from build123d import *

# Parameters (mm, degrees)
OHGC_BASE_DEPTH  = 2.54
SKETCH7_R        = 1.27
SCREWHOLES_DEPTH = 3.54


with BuildPart() as part:
    # Sketch2 → OHGC BASE (new body)
    with BuildSketch(Plane(origin=(0, 0, 0), x_dir=(1, 0, 0), z_dir=(0, 1, 0))):
        with BuildLine():
            Line((12.7, 0), (25.4, 0))
            ThreePointArc((25.4, 0), (34.380256121, 3.719743879), (38.1, 12.7))
            Line((38.1, 12.7), (38.1, 38.1))
            ThreePointArc((38.1, 38.1), (38.996434372, 41.352863652), (41.432636832, 43.68730879))
            Line((41.432636832, 43.68730879), (69.022459682, 58.586881809))
            ThreePointArc((69.022459682, 58.586881809), (73.920701901, 62.034864891), (77.875264971, 66.534064274))
            Line((77.875264971, 66.534064274), (81.475778144, 71.764628765))
            ThreePointArc((81.475778144, 71.764628765), (85.749269843, 82.951996559), (84.42171275, 94.853993098))
            Line((84.42171275, 94.853993098), (66.518139685, 144.04365582))
            ThreePointArc((66.518139685, 144.04365582), (61.868464143, 150.103230962), (54.584043401, 152.4))
            Line((54.584043401, 152.4), (6.35, 152.4))
            ThreePointArc((6.35, 152.4), (1.859871939, 150.540128061), (0, 146.05))
            Line((0, 146.05), (0, 12.7))
            ThreePointArc((0, 12.7), (3.719743879, 3.719743879), (12.7, 0))
        make_face()
    extrude(amount=OHGC_BASE_DEPTH)

    # Sketch7 → Screwholes (cut, through all)
    with BuildSketch(Plane(origin=(0, 0, 0), x_dir=(1, 0, 0), z_dir=(0, 1, 0))):
        with Locations((3.302, 149.098)):
            Circle(SKETCH7_R)
        with Locations((60.719962059, 148.463)):
            Circle(SKETCH7_R)
        with Locations((83.655901234, 83.21908607)):
            Circle(SKETCH7_R)
        with Locations((19.05, 22.352)):
            Circle(SKETCH7_R)
        with Locations((19.05, 2.032)):
            Circle(SKETCH7_R)
    extrude(amount=SCREWHOLES_DEPTH, mode=Mode.SUBTRACT)


solid = part.part
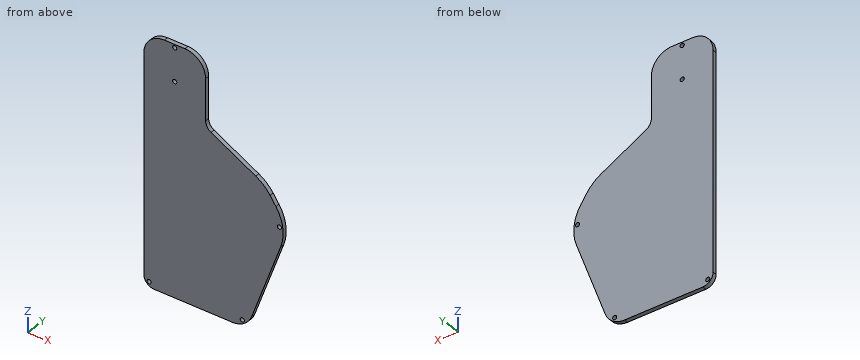
Geometry check sheet. Reference: the model listing, model coordinates, mm. Give positions to 0.01 mm unless a question says otherwise; leave off trailing zeros. Loops run counter-clockwise (first coordinate to the right, second up) from the corner with the lowest first, then second, coordinate; pieces in that order, holes last. Notation, with made-up numbers: (28.25, 60.25) -> (74.25, 60.25) arc R26 cw to (74.25, 95.25) -> close; hole circle Ø4 at (2, 79.25). An arc over 180 degrees is marked (long way). Answer in a Markdown table with one row per item. Add a question column.
1) Gauge pin test, flat end, axial feed: P1, Ø1, axis at x = 58.5, y = 2, coming from the -Z side. Record the tip position at first contact, or that the pin passes through.
2) Cross-section at C-C on x = 45.5. Record the boundary of the cut face in (y, z).
3) Cross-section at B-B on z = -142. Record the boundary of the cut face in (x, y), and give its area (3 significant figures).
4) Cross-section at A-A on y = 0.8. Record the boundary of the cut face in (x, z), and give its area (3 significant figures).
5) Material ranges on probe 1 along Z at (x, y) = (19.05, 2.05); probe 2 along X at (y, z) = (0.45, -13.5); probe 3 along Z at (x, y) = (18, 2.1), recorded low to high. Write a range as from..to.
Outcome:
| question | item | result |
|---|---|---|
| 1 | P1 | stops at z = -151.93 |
| 2 | outline | (0, -152.4) -> (2.54, -152.4) -> (2.54, -45.88) -> (0, -45.88) -> close |
| 3 | outline | (0, 0) -> (67.26, 0) -> (67.26, 2.54) -> (0, 2.54) -> close |
| 3 | area | 171 mm^2 |
| 4 | outline | (0, -146.05) arc R6.35 ccw to (6.35, -152.4) -> (54.58, -152.4) arc R12.7 ccw to (66.52, -144.04) -> (84.42, -94.85) arc R25.4 ccw to (81.48, -71.76) -> (77.88, -66.53) arc R25.4 ccw to (69.02, -58.59) -> (41.43, -43.69) arc R6.35 cw to (38.1, -38.1) -> (38.1, -12.7) arc R12.7 ccw to (25.4, 0) -> (12.7, 0) arc R12.7 ccw to (0, -12.7) -> close; hole circle Ø2.54 at (3.3, -149.1); hole circle Ø2.54 at (19.05, -22.35); hole circle Ø2.54 at (19.05, -2.03); hole circle Ø2.54 at (60.72, -148.46); hole circle Ø2.54 at (83.66, -83.22) |
| 4 | area | 9,600 mm^2 |
| 5 | probe 1 | z = -152.4..-23.62, -21.08..-3.3, -0.76..0 |
| 5 | probe 2 | x = 0..38.1 |
| 5 | probe 3 | z = -152.4..-23.07, -21.64..-2.75, -1.32..0 |
